Part model, mm, in its own coordinate system. A direction names the side the tool comes from. Coordinates: 2 decimals unless noted, no trailing zeros. Order: outer loops, then holes, each group sorted by start corner. A loop starts at its lowest first (then second) coordinate and runs counter-clockwise, first axis right, second up.
Autodesk Inventor part; units mm, degrees
ref_plane "YZ Plane" through (0, 0, 0) normal (1, 0, 0) x (0, 1, 0)
ref_plane "XZ Plane" through (0, 0, 0) normal (0, 1, 0) x (-1, 0, 0)
ref_plane "XY Plane" through (0, 0, 0) normal (0, 0, 1) x (1, 0, 0)
sketch "Sketch1" plane through (0, 0, 0) normal (0, 1, 0) x (-1, 0, 0)
  line L0 (26, 16) -> (-26, 16)
  line L1 (-26, 16) -> (-26, -16)
  line L2 (-26, -16) -> (26, -16)
  line L3 (26, -16) -> (26, 16)
  line L4 (26, 16) -> (-26, -16) construction
  line L5 (-26, 16) -> (26, -16) construction
  point P0 (0, 0)
  dimension "d0" = 52
  dimension "d1" = 32
extrude "Extrusion1" add sketch "Sketch1" along normal blind 2
sketch "Sketch2" plane through (0, 0, 0) normal (0, -1, 0) x (1, 0, 0)
  point P0 (0, 0)
sketch "Sketch3" plane through (0, 0, 0) normal (0, -1, 0) x (1, 0, 0)
  line L0 (-26, 16) -> (26, 16)
  line L1 (-26, -16) -> (-26, 16)
  line L2 (26, -16) -> (-26, -16)
  line L3 (26, 16) -> (26, -16)
  line L4 (24, 14) -> (-24, 14)
  line L5 (-24, 14) -> (-24, -14)
  line L6 (-24, -14) -> (24, -14)
  line L7 (24, -14) -> (24, 14)
  point P0 (0, 0)
  dimension "d4" = 2
extrude "Extrusion2" add sketch "Sketch3" along normal blind 1
sketch "Sketch4" plane through (0, 0, 0) normal (0, -1, 0) x (1, 0, 0)
  point P0 (0, 0)
sketch "Sketch5" plane through (0, 2, 0) normal (0, 1, 0) x (1, 0, 0)
  line L0 (-22, 12) -> (-20, 12)
  line L1 (-20, 12) -> (-20, -12)
  line L2 (-20, -12) -> (-22, -12)
  line L3 (-22, -12) -> (-22, 12)
  line L4 (-26, 16) -> (-26, -16)
  line L5 (26, 16) -> (-26, 16)
  line L6 (-26, -16) -> (26, -16)
  point P0 (0, 0)
  dimension "d7" = 2
  dimension "d8" = 4
  dimension "d9" = 4
  dimension "d10" = 4
extrude "Extrusion3" cut sketch "Sketch5" against normal through all
mirror "Mirror1" about plane through (0, 0, 0) normal (1, 0, 0) of "Extrusion3"
properties part number "5x3holder" material "PET Plastic"
(1) Slice it at A-A, the plane z = 9.5. Give the cut face in (x, y), then the cut area to 3 significant figures.
(2) Slice it at C-C, the plane z = -13. Give the cut face in (x, y).
(3) Pull direction X, two halves, no side cores. Call faces 1 (the face through (26, 0, 0)), 2 (the face through (-21, 1, -12)), 3 (the face through (-26, 0, 0)), 4 (the face through (0, 0, 16)): +X half, -X half, draft (parallel to the pull), parting line (faces both ways), or undercut.
(4) Tool access for faces 5 (the face through (0, 0, 0)), 6 (the face through (21, 1, -12)), 7 (the face through (0, 0, -16)): list every direction of +Z, -Z, +X, -X, +Y, -Y with a clear straight run to the whole face (end or side of a thin tool).
(5) Probe line 1 (X direction, y = 1.4, z = 10); line 2 (X direction, y = -0.5, z = -4); line 3 (Z direction, x = 22, y = -0.5). List the from-to ranges inside material, lowest first.
(6) Drop a flat-ended pin along its axis: pin 1 (8 mm diameter, centred on x = -17, z = 4.5, fed in from -Y). Give the stop position or say it passes through.
(7) Slice it at B-B, the plane y = 1.05. Give the cut face in (x, z), then the cut area to 3 significant figures.
(8) Slice it at D-D, the plane x = 10. Give the cut face in (y, z).
Here are the results:
1. outline: (-26, -1) - (-24, -1) - (-24, 0) - (-22, 0) - (-22, 2) - (-26, 2) - close; (-20, 0) - (20, 0) - (20, 2) - (-20, 2) - close; (22, 0) - (24, 0) - (24, -1) - (26, -1) - (26, 2) - (22, 2) - close
1. area: 100 mm2
2. outline: (-26, -1) - (-24, -1) - (-24, 0) - (24, 0) - (24, -1) - (26, -1) - (26, 2) - (-26, 2) - close
3. face 1: +X half
3. face 2: undercut
3. face 3: -X half
3. face 4: draft
4. face 5: -Y
4. face 6: +Y, -Y
4. face 7: -Z, +X, -X, +Y, -Y
5. line 1: x = -26 to -22, -20 to 20, 22 to 26
5. line 2: x = -26 to -24, 24 to 26
5. line 3: z = -16 to -14, 14 to 16
6. pin 1: stops at y = 0
7. outline: (-26, -16) - (26, -16) - (26, 16) - (-26, 16) - close; hole (-22, -12) - (-20, -12) - (-20, 12) - (-22, 12) - close; hole (20, -12) - (22, -12) - (22, 12) - (20, 12) - close
7. area: 1,570 mm2
8. outline: (-1, -16) - (2, -16) - (2, 16) - (-1, 16) - (-1, 14) - (0, 14) - (0, -14) - (-1, -14) - close
